Design review of the part built by this model. Coordinates are the model's own, in mm. A direction names the side the tool comes from. Coordinates: 2 decimals unless noted, no trailing zeros. Write each loop counter-clockwise with the first axis right and the second up, starting at its lowest first coordinate (ties: lowest second). Pieces come first, ordered by that corner, then holes. Notation, with made-up numbers: (9, 47.5) - (33, 47.5) arc R31 cw to (33, 76.5) - close; hole circle Ø3 at (80.25, -17). An arc over 180 degrees is marked (long way). Use a Markdown table: item, result.
Autodesk Inventor part; units mm, degrees
ref_plane "YZ Plane" through (0, 0, 0) normal (1, 0, 0) x (0, 1, 0)
ref_plane "XZ Plane" through (0, 0, 0) normal (0, 1, 0) x (-1, 0, 0)
ref_plane "XY Plane" through (0, 0, 0) normal (0, 0, 1) x (1, 0, 0)
sketch "Sketch1" plane through (0, 0, 0) normal (0, 1, 0) x (-1, 0, 0)
  line L0 (10.2, -1.85) -> (10.2, 0)
  line L1 (10.2, 0) -> (11.7, 0)
  line L2 (11.7, 0) -> (11.7, -4.35)
  line L3 (11.7, -4.35) -> (0, -4.35)
  line L4 (0, -4.35) -> (0, 0)
  line L5 (0, 0) -> (1.5, 0)
  line L6 (1.5, 0) -> (1.5, -1.85)
  arc A0 (1.5, -1.85) -> (2.5, -2.85) centre (2.5, -1.85) ccw
  line L7 (2.5, -2.85) -> (9.2, -2.85)
  arc A1 (9.2, -2.85) -> (10.2, -1.85) centre (9.2, -1.85) ccw
  line L8 (10.2, 1.85) -> (10.2, 0)
  line L9 (11.7, 0) -> (11.7, 4.35)
  line L10 (11.7, 4.35) -> (0, 4.35)
  line L11 (0, 4.35) -> (0, 0)
  line L12 (1.5, 0) -> (1.5, 1.85)
  arc A2 (2.5, 2.85) -> (1.5, 1.85) centre (2.5, 1.85) ccw
  line L13 (2.5, 2.85) -> (9.2, 2.85)
  arc A3 (10.2, 1.85) -> (9.2, 2.85) centre (9.2, 1.85) ccw
extrude "Extrusion1" add sketch "Sketch1" against normal blind 4 contours L8 A3 L13 A2 L12 L5 L11 L10 L9 L1
sketch "Sketch2" plane through (0, 0, 0) normal (0, 1, 0) x (1, 0, 0)
  line L0 (-0.75, 0) -> (-0.75, 2.63)
  arc A0 (-0.75, 2.63) -> (-1.75, 3.63) centre (-1.75, 2.63) ccw
  line L1 (-1.75, 3.63) -> (-9.95, 3.63)
  arc A1 (-9.95, 3.63) -> (-10.95, 2.63) centre (-9.95, 2.63) ccw
  line L2 (-10.95, 2.63) -> (-10.95, 0)
  line L3 (-10.95, 0) -> (-0.75, 0)
  line L4 (-0.75, 0) -> (-0.75, -2.63)
  arc A2 (-1.75, -3.63) -> (-0.75, -2.63) centre (-1.75, -2.63) ccw
  line L5 (-1.75, -3.63) -> (-9.95, -3.63)
  arc A3 (-10.95, -2.63) -> (-9.95, -3.63) centre (-9.95, -2.63) ccw
  line L6 (-10.95, -2.63) -> (-10.95, 0)
  arc A4 (-7.85, 0) -> (-3.85, 0) centre (-5.85, 0) ccw
  point P0 (0, 0)
  dimension "d2" = 2
extrude "Extrusion2" add sketch "Sketch2" along normal blind 85 contours L4 A2 L5 A3 L6 L3 A4
sketch "Sketch3" plane through (0, 85, 0) normal (0, 1, 0) x (1, 0, 0)
  point P0 (0, 0)
sketch "Sketch4" plane through (-9.95, 0, 3.63) normal (0, 0, 1) x (1, 0, 0)
  circle A0 centre (7, 90) radius 10
  line L0 (-1.75, 0) -> (9.95, 0)
  line L1 (9.2, 0) -> (9.2, 85)
  line L2 (-1, 0) -> (-1, 85)
  dimension "d6" = 20
  dimension "d12" = 90
  dimension "d14" = 8
extrude "Extrusion3" add sketch "Sketch4" against normal up to surface (3.63 mm away) contours A0
sketch "Sketch5" plane through (-9.95, 0, 3.63) normal (0, 0, 1) x (1, 0, 0)
  circle A0 centre (7, 90) radius 1.7
  circle A1 centre (7, 90) radius 10
  point P0 (9.95, 0)
  point P1 (0, 82.8586)
  point P2 (8.2, 80.0723)
  dimension "d9" = 3.4
extrude "Extrusion4" cut sketch "Sketch5" against normal blind 120 contours A0
properties part number "microphone2"
(1) For pin 1 (0.6 mm diameter, centred on y = -1.5, z = 1.5, fed in from -X); pin 2 (4.5 mm diameter, centred on x = -6.5, y = -3, fed in from -Z); pin 3 (0.6 mm diameter, centred on y = -2, z = 0.5, fed in from +X), all flat-tipped, find the tip position at first contact; note any pin that passes through.
Determined:
| item | result |
|---|---|
| pin 1 | x = -11.7 |
| pin 2 | z = 2.85 |
| pin 3 | x = 0 |
(2) Take a section at A-A on y = 90. Write out the cut boundary in (x, z), and give its area (3 significant figures).
Determined:
| item | result |
|---|---|
| outline | (-12.95, 0) - (-4.65, 0) - (-4.65, 3.63) - (-12.95, 3.63) - close; (-1.25, 0) - (7.05, 0) - (7.05, 3.63) - (-1.25, 3.63) - close |
| area | 60.3 mm2 |
(3) For L1, parallel to X at y = 90, z = 1.9; L2, parallel to Y at x = -2.95, z = 2.2; L3, parallel to Z at x = -9, y = 29.5, list the stretches that pass through material, from the lowest coordinate up. Write a range as from..to.
Determined:
| item | result |
|---|---|
| L1 | -12.95..-4.65, -1.25..7.05 |
| L2 | 0..88.3, 91.7..100 |
| L3 | 0..3.63 |
(4) Machinability: for faces 4 (the flat face through (-5, 62, 3.63)), 5 (the flat face through (-6, 0, 4)), 6 (the flat face through (-10.2, -2, 1)), which of the approach directions +Z, -Z, +X, -X, +Y, -Y give a long, thin tool a straight path to every point of the face, cutting with its end or side? Answer none if there is none.
Determined:
| item | result |
|---|---|
| face 4 | +Z, +X, -X, +Y |
| face 5 | +Z |
| face 6 | -Z, -Y |
(5) Take a section at D-D on y = 5.5. Write out the cut boundary in (x, z).
Determined:
| item | result |
|---|---|
| outline | (-10.95, 0) - (-7.85, 0) arc R2 cw to (-3.85, 0) - (-0.75, 0) - (-0.75, 2.63) arc R1 ccw to (-1.75, 3.63) - (-9.95, 3.63) arc R1 ccw to (-10.95, 2.63) - close |
(6) Draft analysis for pull direction Y (two halves, no side actions). For faces 1 (the flat face through (-10.95, 41, 1)), 2 (the flat face through (-6, -2, 4.35)), 3 (the flat face through (-5.9, 0, 2.4)), state which applies: +Y half, -Y half, draft (parallel to the pull), parting line (faces both ways), or undercut.
Determined:
| item | result |
|---|---|
| face 1 | undercut |
| face 2 | draft |
| face 3 | -Y half |
(7) Take a section at C-C on x = -5.85. Write out the cut boundary in (y, z), and give its area (3 significant figures).
Determined:
| item | result |
|---|---|
| outline | (-4, 2.85) - (0, 2.85) - (0, 2) - (80.43, 2) - (80.43, 0) - (99.57, 0) - (99.57, 3.63) - (0, 3.63) - (0, 4.35) - (-4, 4.35) - close |
| area | 207 mm2 |
(8) Take a section at B-B on z = 0.95. Write out the cut boundary in (x, y) (3 decimals), and give its area (3 significant figures).
Determined:
| item | result |
|---|---|
| outline | (-11.7, -4) - (-10.2, -4) - (-10.2, 0) - (-7.61, 0) - (-7.61, 81.152) arc R10 ccw to (-4.09, 80.065) - (-4.09, 0) - (-1.5, 0) - (-1.5, -4) - (0, -4) - (0, 0) - (-0.75, 0) - (-0.75, 80.245) arc R10 ccw (long way) to (-10.95, 84) - (-10.95, 0) - (-11.7, 0) - close; hole circle Ø3.4 at (-2.95, 90) |
| area | 860 mm2 |
